Verification items for this drawing (mm, ordinates from the low corner). Coordinates: 2 decimals unless noted, no trailing zeros. Loops run counter-clockwise (first coordinate to the right, second up) from the corner with the lowest first, then second, coordinate; pieces in that order, holes last. Notation, with made-up numbers: (63, 20.25) - (81, 20.25) arc R7 ccw to (81, 24.25) - close; hole circle Ø4 at (69, 52.25). An arc over 180 degrees is marked (long way). One line per item, written item: value. Start each with the question number.
(1) Section check A-A (y = 7.5). Record the boundary of the cut face in (x, z).
(2) Thickness scan on probe 1 along Z at (x, y) = (4.5, 8.65); probe 2 along X at (y, z) = (1.5, 33). Record the ranges inside material, lowest first. Write a range as [from, to].
(3) Section check D-D (z = 33). Record the boundary of the cut face in (x, y), plus the area to 3 significant figures.
(4) Section check C-C (z = 52.5). Record the boundary of the cut face in (x, y), plus the area to 3 significant figures.
(5) Gauge pin test, flat end, axial feed: P1, Ø2.5, axis at x = 4.5, z = 3.5, coming from the +Y side. Record the tip position at first contact, or that the pin passes through.
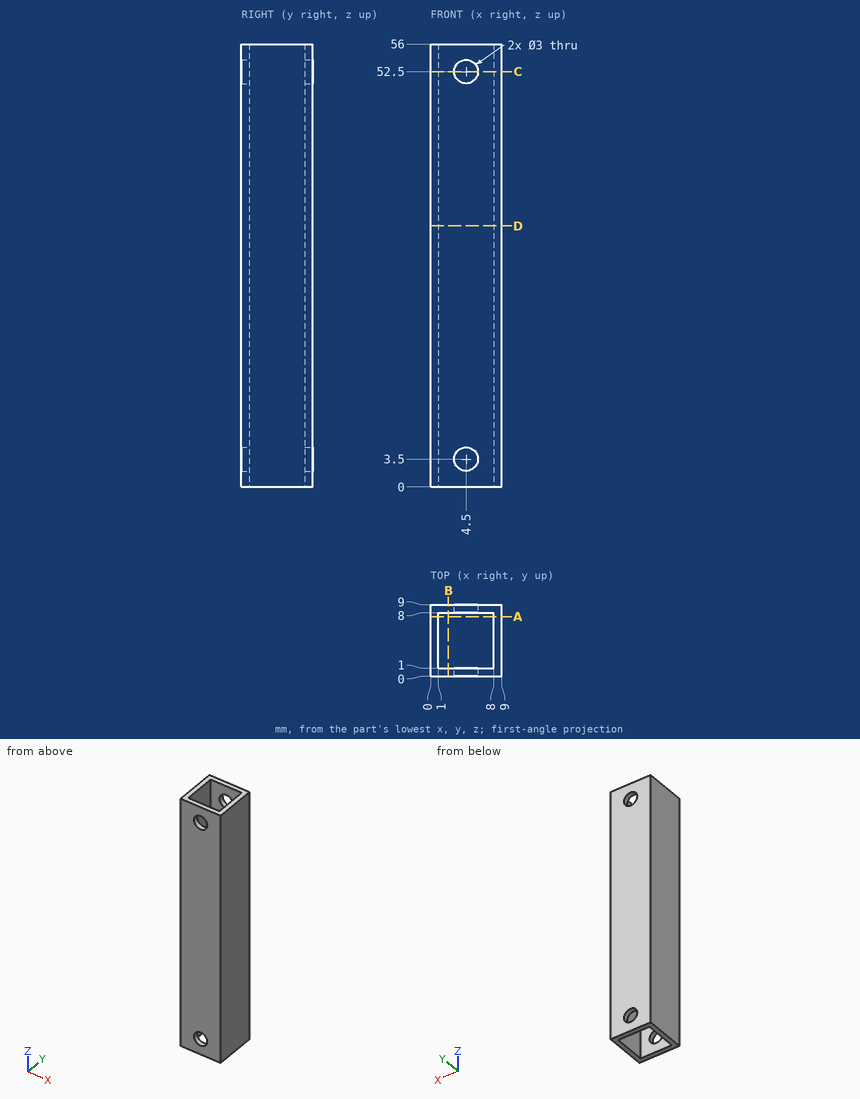
Responses:
1. outline: (0, 0) - (1, 0) - (1, 56) - (0, 56) - close; (8, 0) - (9, 0) - (9, 56) - (8, 56) - close
2. probe 1: z = [0, 2], [5, 51], [54, 56]
2. probe 2: x = [0, 1], [8, 9]
3. outline: (0, 0) - (9, 0) - (9, 9) - (0, 9) - close; hole (1, 1) - (8, 1) - (8, 8) - (1, 8) - close
3. area: 32.0 mm²
4. outline: (0, 0) - (3, 0) - (3, 1) - (1, 1) - (1, 8) - (3, 8) - (3, 9) - (0, 9) - close; (6, 0) - (9, 0) - (9, 9) - (6, 9) - (6, 8) - (8, 8) - (8, 1) - (6, 1) - close
4. area: 26.0 mm²
5. P1: passes through
